Input: part model. Units: mm. Frame: model coordinates. Face numbers are marked on the shaded views. A direction names the side the tool comes from. Coordinates: 2 decimals unless noted, no trailing zeros. Order: outer loops, then holes, each group sorted by start corner. A loop starts at its lowest first (then second) coordinate and runs counter-clockwise, first axis right, second up. Notation, with made-up numbers: (45.25, 0.25) - (61.25, 0.25) arc R21 cw to (61.25, 16.25) - close; hole circle Ø11 at (-19.5, 74.25). An arc over 180 degrees is marked (long way). One line per question, with ' | ' between items.
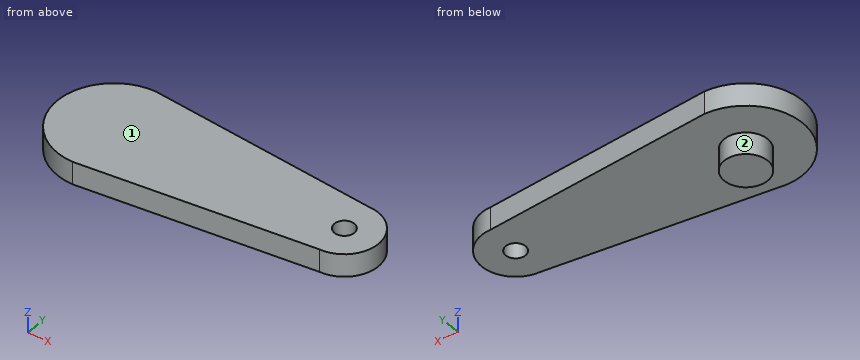
from build123d import *

# Parameters (mm, degrees)
PAD_DEPTH    = 25
SKETCH001_R  = 48
PAD001_DEPTH = 48
SKETCH002_R  = 22
POCKET_DEPTH = 51


with BuildPart() as part:
    # Sketch → Pad (new body, symmetric)
    with BuildSketch(Plane.XY):
        with BuildLine():
            ThreePointArc((0, 125), (-125, 0), (0, -125))
            Line((0, -125), (500, -75))
            ThreePointArc((500, -75), (575, 0), (500, 75))
            Line((0, 125), (500, 75))
        make_face()
    extrude(amount=PAD_DEPTH, both=True)

    # Sketch001 (on Face5 of Pad) → Pad001 (join)
    with BuildSketch(Plane(origin=(0, 0, -25), x_dir=(1, 0, 0), z_dir=(0, 0, -1))):
        Circle(SKETCH001_R)
    extrude(amount=PAD001_DEPTH)

    # Sketch002 (on Face5 of Pad001) → Pocket (cut)
    with BuildSketch(Plane.XY.offset(25)):
        with Locations((500, 0)):
            Circle(SKETCH002_R)
    extrude(amount=-POCKET_DEPTH, mode=Mode.SUBTRACT)


solid = part.part
Item 1: Ray query, line 1 (Y direction, x = 500, z = -8); line 2 (Z direction, x = 472, y = -11.5); line 3 (X direction, y = -14.5, z = -17). Return the intervals inside material, ascending.
Data:
line 1: -75 to -22, 22 to 75 | line 2: -25 to 25 | line 3: -124.16 to 483.45, 516.55 to 573.58
Item 2: Section B-B on z = 4. Return the cut outline in (x, y).
Data:
outline: (0, -125) - (500, -75) arc R75 ccw to (500, 75) - (0, 125) arc R125 ccw to start; hole circle Ø44 at (500, 0)
Item 3: Access query for the marked faces 1 and 2. Directions: +Z, -Z, +X, -X, +Y, -Y. A direction counts if a zero-diameter tool reaches every point of the face in a straight line with its end or side. Return the directions, or none.
Data:
face 1: +Z, +X, -X, +Y, -Y | face 2: -Z
Item 4: Section D-D on z = -36.5. Return the cut outline in (x, y).
Data:
outline: circle Ø96 at (0, 0)
Item 5: Section A-A on y = 0. Return the cut outline in (x, z), and give its area (3 significant figures).
Data:
outline: (-125, -25) - (-48, -25) - (-48, -73) - (48, -73) - (48, -25) - (478, -25) - (478, 25) - (-125, 25) - close; (522, -25) - (575, -25) - (575, 25) - (522, 25) - close | area: 37,400 mm^2
Item 6: Section C-C on x = -8. Return the cut outline in (y, z).
Data:
outline: (-124.74, -25) - (-47.33, -25) - (-47.33, -73) - (47.33, -73) - (47.33, -25) - (124.74, -25) - (124.74, 25) - (-124.74, 25) - close
Item 7: Contact query for flat-ended pins moving along their axis: P1, Ø10, axis at x = 438.5, z = -0.5, coming from the +Y side; P2, Ø12, axis at y = -16.5, z = -24.5, coming from the +X side; P3, Ø4, axis at x = 482, z = -17, coming from the -Y side. Output: stop coordinate, or through.
Data:
P1: y = 81.65 | P2: x = 574.26 | P3: y = -77
